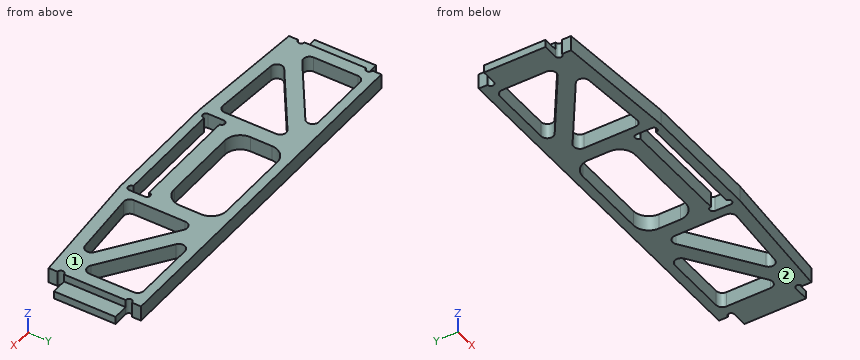
Autodesk Inventor part; units mm, degrees
ref_plane "YZ Plane" through (0, 0, 0) normal (1, 0, 0) x (0, 1, 0)
ref_plane "XZ Plane" through (0, 0, 0) normal (0, 1, 0) x (-1, 0, 0)
ref_plane "XY Plane" through (0, 0, 0) normal (0, 0, 1) x (1, 0, 0)
sketch "スケッチ1" plane through (0, 0, 0) normal (0, 0, 1) x (1, 0, 0)
  line L0 (-59.5, -15) -> (59.5, -15) construction
  line L1 (59.5, -15) -> (59.5, 15) construction
  line L2 (59.5, 15) -> (-59.5, 15) construction
  line L3 (-59.5, 15) -> (-59.5, -15) construction
  line L4 (-59.5, -15) -> (59.5, 15) construction
  line L5 (59.5, -15) -> (-59.5, 15) construction
  line L6 (-59.5, 12.1) -> (-59.5, 15)
  line L7 (-59.5, 15) -> (59.5, 15)
  line L8 (59.5, 15) -> (59.5, 12.1)
  line L9 (-59.5, -12.1) -> (-59.5, -15)
  line L10 (59.5, -15) -> (59.5, -12.1)
  line L11 (-59.5, 10) -> (-64.5, 10)
  line L12 (-64.5, 10) -> (-64.5, -10)
  line L13 (-64.5, -10) -> (-59.5, -10)
  arc A0 (-59.5, 10) -> (-59.5, 12.1) centre (-59.5, 11.05) ccw
  line L14 (0, 0) -> (0, 15) construction
  line L15 (0, 0) -> (-59.5, 0) construction
  arc A1 (-59.5, -12.1) -> (-59.5, -10) centre (-59.5, -11.05) ccw
  line L16 (59.5, 10) -> (64.5, 10)
  line L17 (64.5, 10) -> (64.5, -10)
  line L18 (64.5, -10) -> (59.5, -10)
  arc A2 (59.5, 12.1) -> (59.5, 10) centre (59.5, 11.05) ccw
  arc A3 (59.5, -10) -> (59.5, -12.1) centre (59.5, -11.05) ccw
  line L19 (-59.5, -15) -> (-19.5, -18)
  line L20 (-19.5, -18) -> (19.5, -18)
  line L21 (19.5, -18) -> (59.5, -15)
  line L22 (-19.5, -10) -> (19.5, -10) construction
  line L23 (19.5, -10) -> (19.5, -15) construction
  line L24 (19.5, -15) -> (-19.5, -15) construction
  line L25 (-19.5, -15) -> (-19.5, -10) construction
  line L26 (19.55, -9.95) -> (-19.55, -9.95)
  line L27 (-19.55, -9.95) -> (-19.55, -15.05)
  line L28 (-19.55, -15.05) -> (19.55, -15.05)
  line L29 (19.55, -15.05) -> (19.55, -9.95)
  circle A4 centre (-18.5, -9.95) radius 1.05
  circle A5 centre (-18.5, -15.05) radius 1.05
  circle A6 centre (18.5, -9.95) radius 1.05
  circle A7 centre (18.5, -15.05) radius 1.05
  dimension "d9" = 2.1
  dimension "d0" = 119
  dimension "d1" = 30
  dimension "d2" = 1.05
  dimension "d3" = 20
  dimension "d4" = 5
  dimension "d5" = 5
  dimension "d6" = 0.05
  dimension "d7" = 39
  dimension "d8" = 3
extrude "押し出し1" add sketch "スケッチ1" along normal blind 5
sketch "スケッチ2" plane through (0, 0, 5) normal (0, 0, 1) x (1, 0, 0)
  line L0 (59.5, 12.1) -> (59.5, 15)
  line L1 (-59.5, 15) -> (-59.5, 12.1)
  line L2 (65.6261, 13.972) -> (59.5, 13.972)
  line L3 (59.5, 13.972) -> (59.5, -16.1)
  line L4 (59.5, -16.1) -> (65.6261, -16.1)
  line L5 (65.6261, -16.1) -> (65.6261, 13.972)
  line L6 (-65.8886, -16.1) -> (-59.5, -16.1)
  line L7 (-59.5, -16.1) -> (-59.5, 18.3327)
  line L8 (-59.5, 18.3327) -> (-65.8886, 18.3327)
  line L9 (-65.8886, 18.3327) -> (-65.8886, -16.1)
  point P0 (0, 0)
extrude "押し出し2" cut sketch "スケッチ2" against normal blind 2.5
sketch "スケッチ8" plane through (0, 0, 5) normal (0, 0, 1) x (1, 0, 0)
  line L0 (59.5, 15) -> (-59.5, 15)
  line L1 (-59.5, 10) -> (-59.5, -10)
  line L2 (-59.5, -15) -> (-19.5, -18)
  line L3 (17.45, -15.05) -> (-17.45, -15.05)
  arc A0 (-19.55, -15.05) -> (-17.45, -15.05) centre (-18.5, -15.05) ccw
  line L4 (-19.55, -15.05) -> (-19.55, -9.95)
  arc A1 (-17.45, -9.95) -> (-19.55, -9.95) centre (-18.5, -9.95) ccw
  line L5 (-17.45, -9.95) -> (17.45, -9.95)
  arc A2 (19.55, -9.95) -> (17.45, -9.95) centre (18.5, -9.95) ccw
  line L6 (19.55, -9.95) -> (19.55, -15.05)
  arc A3 (17.45, -15.05) -> (19.55, -15.05) centre (18.5, -15.05) ccw
  line L7 (-55.5, 12) -> (-22.5, 12) construction
  line L8 (-22.5, 12) -> (-22.5, -13.7638) construction
  line L9 (-22.5, -13.7638) -> (-55.5, -11.2888) construction
  line L10 (-55.5, -11.2888) -> (-55.5, 12) construction
  line L11 (17.5013, -10) -> (-17.5013, -10) construction
  arc A4 (-17.5013, -10) -> (-19.5, -9.95) centre (-18.5, -9.95) ccw construction
  line L12 (-19.5, -9.95) -> (-19.5, -15.05) construction
  arc A5 (-19.5, -15.05) -> (-17.5013, -15) centre (-18.5, -15.05) ccw construction
  line L13 (-17.5013, -15) -> (17.5013, -15) construction
  arc A6 (17.5013, -15) -> (19.5, -15.05) centre (18.5, -15.05) ccw construction
  line L14 (19.5, -15.05) -> (19.5, -9.95) construction
  arc A7 (19.5, -9.95) -> (17.5013, -10) centre (18.5, -9.95) ccw construction
  line L15 (-17.5, 12) -> (17.5, 12)
  line L16 (17.5, 12) -> (17.5, -5)
  line L17 (17.5, -5) -> (-17.5, -5)
  line L18 (-17.5, -5) -> (-17.5, 12)
  line L19 (0, 0) -> (0, 15) construction
  line L20 (-22.5, 12) -> (-55.5, -11.2888) construction
  line L21 (-55.5, 12) -> (-26.8358, 12)
  line L22 (-26.8358, 12) -> (-55.5, -8.2289)
  line L23 (-55.5, -8.2289) -> (-55.5, 12)
  line L24 (-51.5807, -11.5827) -> (-22.5, -13.7638)
  line L25 (-22.5, -13.7638) -> (-22.5, 8.9401)
  line L26 (-22.5, 8.9401) -> (-51.5807, -11.5827)
  line L27 (55.5, 12) -> (22.5, 12) construction
  line L28 (22.5, 12) -> (22.5, -13.7638) construction
  line L29 (22.5, -13.7638) -> (55.5, -11.2888) construction
  line L30 (55.5, -11.2888) -> (55.5, 12) construction
  line L31 (22.5, 12) -> (55.5, -11.2888) construction
  line L32 (55.5, 12) -> (26.8358, 12)
  line L33 (26.8358, 12) -> (55.5, -8.2289)
  line L34 (55.5, -8.2289) -> (55.5, 12)
  line L35 (51.5807, -11.5827) -> (22.5, -13.7638)
  line L36 (22.5, -13.7638) -> (22.5, 8.9401)
  line L37 (22.5, 8.9401) -> (51.5807, -11.5827)
  dimension "d51" = 4
  dimension "d52" = 3
  dimension "d53" = 0.05
  dimension "d54" = 3
  dimension "d55" = 4
  dimension "d56" = 5
  dimension "d57" = 5
  dimension "d58" = 5
extrude "押し出し6" cut sketch "スケッチ8" against normal blind 10 contours L15 L16 L17 L18 | L21 L22 L23 | L26 L25 L24 | L34 L33 L32 | L35 L36 L37
fillet "フィレット4" radius 2 12 edges at (-55.5, 12, 2.5) (-55.5, -8.2289, 2.5) (-26.8358, 12, 2.5) (-22.5, 8.9401, 2.5) (-51.5807, -11.5827, 2.5) (-22.5, -13.7638, 2.5) (22.5, 8.9401, 2.5) (26.8358, 12, 2.5) (55.5, -8.2289, 2.5) (55.5, 12, 2.5) (22.5, -13.7638, 2.5) (51.5807, -11.5827, 2.5)
fillet "フィレット4" radius 5 4 edges at (-17.5, -5, 2.5) (-17.5, 12, 2.5) (17.5, 12, 2.5) (17.5, -5, 2.5)
properties part number "コックピット_サブフレーム_1_6" material "アセタール樹脂、黒"
Geometry: final body of the model. Coordinates: model frame, mm. Face numbers are marked on the shaded views. Coordinates: 2 decimals unless noted, no trailing zeros. Order: outer loops, then holes, each group sorted by start corner. A loop starts at its lowest first (then second) coordinate and runs counter-clockwise, first axis right, second up. Notation, with made-up numbers: M 61.5,37.5 L 111.5,37.5 A16 cw 111.5,63.5 Z; hole C 83.25,12.5 d8. An arc over 180 degrees is marked long. Answer in a Markdown table with one row per item. Add a question column.
Q1. Line query: L1, parallel to Y at x = 7.5, z = 2.2; L2, parallel to X at y = -1, z = 4.25; L3, parallel to X at y = -2, z = 2.9. Output: solid intervals per line, ascending.
Q2. Mould query, pull axis Z, two halves, no side actions, for the marked faces 1 and 2. Classes: released by +Z, released by -Z, zero draft, split by the parting line, or undercut.
Q3. Section query A-A on x = -43.5. Return the cut outline in (y, z), and give its area (3 significant figures).
Q4. Contact query for flat-ended pins moving along their axis: P1, Ø3, axis at y = 14, z = 2.5, coming from the -X side; P2, Ø1.5, axis at x = -62, y = -2.5, coming from the +Z side; P3, Ø1.2, axis at y = -2, z = 3.5, coming from the +X side. Output: stop coordinate, or through.
Completed:
| question | item | result |
|---|---|---|
| 1 | L1 | y = -18 to -15.05, -9.95 to -5, 12 to 15 |
| 1 | L2 | x = -59.5 to -55.5, -45.26 to -36.59, -22.5 to -17.4, 17.4 to 22.5, 36.59 to 45.26, 55.5 to 59.5 |
| 1 | L3 | x = -59.5 to -55.5, -46.67 to -38, -22.5 to -17.08, 17.08 to 22.5, 38 to 46.67, 55.5 to 59.5 |
| 2 | face 1 | released by +Z |
| 2 | face 2 | released by -Z |
| 3 | outline | M -16.2,0 L -12.19,0 L -12.19,5 L -16.2,5 Z; M -5.88,0 L 0.24,0 L 0.24,5 L -5.88,5 Z; M 12,0 L 15,0 L 15,5 L 12,5 Z |
| 3 | area | 65.7 mm2 |
| 4 | P1 | stops at x = -59.5 |
| 4 | P2 | stops at z = 2.5 |
| 4 | P3 | stops at x = 59.5 |
